Verification items for the finished model (mm, model axes). A direction names the side the tool comes from. Give positions to 0.01 mm unless a question says otherwise; leave off trailing zeros. Loops run counter-clockwise (first coordinate to the right, second up) from the corner with the lowest first, then second, coordinate; pieces in that order, holes last. Notation, with made-up numbers: (10.25, 19.5) -> (16.25, 19.5) arc R18 cw to (16.25, 51.5) -> close; hole circle Ø2 at (49, 57). An arc over 180 degrees is marked (long way). Use one line per item in the form item = value. Start each with the question number.
from build123d import *

# Parameters (mm, degrees)
EXTRUDE_1_DEPTH     = 7
SKETCH_2_R          = 1.5
CUT_EXTRUDE_1_DEPTH = 50
SKETCH_5_R          = 2
EXTRUDE_2_DEPTH     = 2
FILLET_2_R          = 2
SKETCH_3_R          = 1.5
EXTRUDE_3_DEPTH     = 12


with BuildPart() as part:
    # 草图1 → 凸台-拉伸1 (new body)
    with BuildSketch(Plane.XY):
        with BuildLine():
            Line((0, 13.97371149), (0, 0))
            Line((0, 0), (8, 0))
            Line((8, 0), (8, 7))
            ThreePointArc((8, 7), (8.585786438, 8.414213562), (10, 9))
            Line((10, 9), (27, 9))
            ThreePointArc((27, 9), (28.414213562, 8.414213562), (29, 7))
            Line((29, 7), (29, 0))
            Line((29, 0), (37, 0))
            Line((37, 0), (37, 13.97371149))
            ThreePointArc((37, 13.97371149), (36.897888614, 14.979040852), (36.59572515, 15.943307983))
            Line((36.59572515, 15.943307983), (34.317232535, 21.259790752))
            ThreePointArc((34.317232535, 21.259790752), (34.062511941, 22.01564259), (33.93122444, 22.802381539))
            Line((33.93122444, 22.802381539), (31, 57))
            Line((31, 57), (24.5, 57))
            Line((24.5, 57), (24.5, 34))
            ThreePointArc((24.5, 34), (23.914213562, 32.585786438), (22.5, 32))
            Line((22.5, 32), (18.5, 32))
            Line((18.5, 32), (14.5, 32))
            ThreePointArc((14.5, 32), (13.085786438, 32.585786438), (12.5, 34))
            Line((12.5, 34), (12.5, 57))
            Line((12.5, 57), (6, 57))
            Line((6, 57), (3.06877556, 22.802381539))
            ThreePointArc((3.06877556, 22.802381539), (2.937488059, 22.01564259), (2.682767465, 21.259790752))
            Line((2.682767465, 21.259790752), (0.40427485, 15.943307983))
            ThreePointArc((0.40427485, 15.943307983), (0.102111386, 14.979040852), (0, 13.97371149))
        make_face()
        Polygon((6, 13.736227722), (10.229385492, 25.248189223), (14.834170093, 15), align=None, mode=Mode.SUBTRACT)
        Polygon((23.922560752, 15), (19.317776151, 25.248189223), (29, 27.065867355), (29, 15), align=None, mode=Mode.SUBTRACT)
    extrude(amount=EXTRUDE_1_DEPTH)

    # 草图2 → 切除-拉伸1 (cut, symmetric)
    with BuildSketch(Plane(origin=(8, 0, 0), x_dir=(0, 0, -1), z_dir=(1, 0, 0))):
        with Locations(Location((-3.5, 2, 0), (0, 0, 180))):
            Circle(SKETCH_2_R)
    extrude(amount=CUT_EXTRUDE_1_DEPTH, both=True, mode=Mode.SUBTRACT)

    # 草图5 → 凸台-拉伸2 (add)
    with BuildSketch(Plane.ZY.offset(-3)):
        with Locations((3.5, 32)):
            Circle(SKETCH_5_R)
    extrude(amount=-EXTRUDE_2_DEPTH)

    # 草图6 → 旋转1 (revolve)
    with BuildSketch(Plane(origin=(0, 0, 3.5), x_dir=(-1, 0, 0), z_dir=(0, 0, -1)), mode=Mode.PRIVATE) as revolve_1_sk:
        with BuildLine():
            Line((-3, 32), (-3, 30))
            Line((-3, 30), (-2.237436867, 30.762563133))
            ThreePointArc((-2.237436867, 30.762563133), (-0.330303993, 30.383210818), (0.75, 32))
            Line((0.75, 32), (-1, 32))
            Line((-1, 32), (-3, 32))
        make_face()
    revolve(revolve_1_sk.sketch.rotate(Axis((3, 32, 3.5), (-1, 0, 0)), 270), axis=Axis((3, 32, 3.5), (-1, 0, 0)))

    # 圆角2
    fillet_2_edges = [part.edges().sort_by_distance(p)[0] for p in [
        (33, 0, 0),
        (4, 0, 0),
        (4, 0, 7),
        (33, 0, 7),
    ]]
    fillet(fillet_2_edges, radius=FILLET_2_R)

    # 草图3 → 凸台-拉伸3 (add)
    with BuildSketch(Plane(origin=(12.5, 0, 0), x_dir=(0, 0, -1), z_dir=(1, 0, 0))):
        with Locations(Location((-3.5, 54, 0), (0, 0, 90))):
            Circle(SKETCH_3_R)
    extrude(amount=EXTRUDE_3_DEPTH)


solid = part.part
Item 1: Material ranges on line 1 (X direction, y = 4.5, z = 1.25); line 2 (X direction, y = 18.5, z = 2); line 3 (Z direction, x = 2.5, y = 2), recorded low to high.
Item 2: Sectioned sample at D-D, the plane y = 54. Enter the section's corners in (x, z).
Item 3: Gauge pin test, flat ends, axial feed: pin 1 Ø1 at (y, z) = (33, 3) entering from +X; pin 2 Ø2 at (y, z) = (19.5, 4.5) entering from -X; pin 3 Ø3.5 at (y, z) = (2, 3) entering from -X. Record the tip position at first contact, or that the pin passes through.
Item 4: Draft check along X on faces 1 (the flat face through (18, 9, 3)), 2 (the flat face through (4.555, 40.141, 3.451)), 3 (the cylindrical face through (33.06, 0.6, 0.57)). Enter one of: +X half, -X half, draft (parallel to the pull), parting line (faces both ways), or undercut.
Item 5: Sectioned sample at B-B, the plane x = 20.5. Enter the section's corners in (y, z).
Item 6: Sectioned sample at A-A, the plane y = 22. Enter the section's corners in (x, z).
Item 7: Sectioned sample at C-C, the plane y = 42.5. Enter the section's corners in (x, z), and give its area (3 significant figures).
Item 8: Tool access check on faces 4 (the cylindrical face through (18.42, 55.43, 3.95)), 5 (the cylindrical face through (3.406, 33.686, 4.575)), 6 (the cylindrical face through (0.105, 14.993, 3.451)), 7 (the flat face through (24.091, 26.144, 3.451)), 8 (the cylindrical face through (33.06, 0.6, 6.43)). Record the directions out of +Z, -Z, +X, -X, +Y, -Y that give a thin tool (end or side, any length) a straight path to the whole face; none if there is none.
Outcome:
q1.line_1 = 0 to 8, 29 to 37
q1.line_2 = 1.5 to 7.75, 13.26 to 22.35, 29 to 35.5
q1.line_3 = 0 to 2, 5 to 7
q2.outline = (5.74, 0) -> (12.5, 0) -> (12.5, 2) -> (24.5, 2) -> (24.5, 0) -> (31.26, 0) -> (31.26, 7) -> (24.5, 7) -> (24.5, 5) -> (12.5, 5) -> (12.5, 7) -> (5.74, 7) -> close
q3.pin_1 = 33.1
q3.pin_2 = 1.5
q3.pin_3 = 0
q4.face_1 = undercut
q4.face_2 = -X half
q4.face_3 = draft
q5.outline = (9, 0) -> (22.62, 0) -> (22.62, 7) -> (9, 7) -> close; (25.47, 0) -> (32, 0) -> (32, 7) -> (25.47, 7) -> close; circle Ø3 at (54, 3.5)
q6.outline = (2.93, 0) -> (9.04, 0) -> (9.04, 7) -> (2.93, 7) -> close; (11.69, 0) -> (20.78, 0) -> (20.78, 7) -> (11.69, 7) -> close; (29, 0) -> (34.07, 0) -> (34.07, 7) -> (29, 7) -> close
q7.outline = (4.76, 0) -> (12.5, 0) -> (12.5, 7) -> (4.76, 7) -> close; (24.5, 0) -> (32.24, 0) -> (32.24, 7) -> (24.5, 7) -> close
q7.area = 108 mm^2
q8.face_4 = none
q8.face_5 = -X
q8.face_6 = +Z, -Z, -X
q8.face_7 = +Z, -Z
q8.face_8 = +Z, +X, -X, -Y
